```python
from build123d import *

# Parameters (mm, degrees)
F0_W           = 100
F0_H           = 70
F1_DEPTH       = 200
F2_R           = 25
F3_T           = -25
F5_START       = -25
F5_DEPTH       = 50
F6_R           = 24.99999
F9_D           = 25
F9_DEPTH       = 100
F9_TIP         = 7.5107577378
F9_ON_F8_D     = 25
F9_ON_F8_DEPTH = 100
F9_ON_F8_TIP   = 7.5107577378
F10_R          = 15
F11_DEPTH      = 50


# Not quite as in the source:
# - a fillet or chamfer is up to 0.001 mm smaller than in the source, because OpenCascade refuses the exact size


with BuildPart() as f1:
    # F0 (on Front) → F1 (new body)
    with BuildSketch(Plane.XZ):
        with Locations((50, -35)):
            Rectangle(F0_W, F0_H)
    extrude(amount=-F1_DEPTH)

    # F2
    f2_edges = [f1.edges().sort_by_distance(p)[0] for p in [
        (100, 100, -70),
        (0, 100, -70),
        (100, 200, -35),
        (0, 200, -35),
    ]]
    fillet(f2_edges, radius=F2_R)

    # F3
    f3_openings = [f1.faces().sort_by_distance(p)[0] for p in [
        (100, 87.5, -22.5),
        (50, 200, -35),
        (92.67767, 192.67767, -35),
        (7.32233, 192.67767, -35),
        (0, 87.5, -22.5),
        (92.67767, 100, -62.67767),
        (50, 100, -70),
        (7.32233, 100, -62.67767),
    ]]
    offset(amount=F3_T, openings=f3_openings)

    # F4 (on face) → F5 (join)
    with BuildSketch(Plane.YZ.offset(100).offset(F5_START)):
        Polygon((17.6776695297, 17.6776695297), (0, 0), (163, 0), (81.5, 81.5), (28.2842712475, 28.2842712475), (38.8908729653, 17.6776695297), (28.2842712475, 7.0710678119), align=None)
    extrude(amount=-F5_DEPTH)

    # F6 (radius 25 in the source; OpenCascade refuses exactly that, so slightly less here)
    f6_edges = [f1.edges().sort_by_distance(p)[0] for p in [
        (75, 122.25, 40.75),
        (25, 122.25, 40.75),
    ]]
    fillet(f6_edges, radius=F6_R)

    # F9
    with Locations(Plane.XZ):
        with Locations((75, -45), (25, -45)):
            Hole(F9_D / 2, depth=F9_DEPTH)
            with Locations((0, 0, -(F9_DEPTH + F9_TIP / 2))):  # 118° drill point
                Cone(0, F9_D / 2, F9_TIP, mode=Mode.SUBTRACT)

    # F9 on F8
    with Locations(Plane.XY):
        with Locations((75, 175), (25, 175)):
            Hole(F9_ON_F8_D / 2, depth=F9_ON_F8_DEPTH)
            with Locations((0, 0, -(F9_ON_F8_DEPTH + F9_ON_F8_TIP / 2))):  # 118° drill point
                Cone(0, F9_ON_F8_D / 2, F9_ON_F8_TIP, mode=Mode.SUBTRACT)

    # F10 (on face) → F11 (cut)
    with BuildSketch(Plane(origin=(0, 0, 0), x_dir=(1, 0, 0), z_dir=(0, -0.7071067812, 0.7071067812))):
        with Locations((50, 90.2584053334)):
            Circle(F10_R)
    extrude(amount=-F11_DEPTH, mode=Mode.SUBTRACT)


solid = f1.part
```
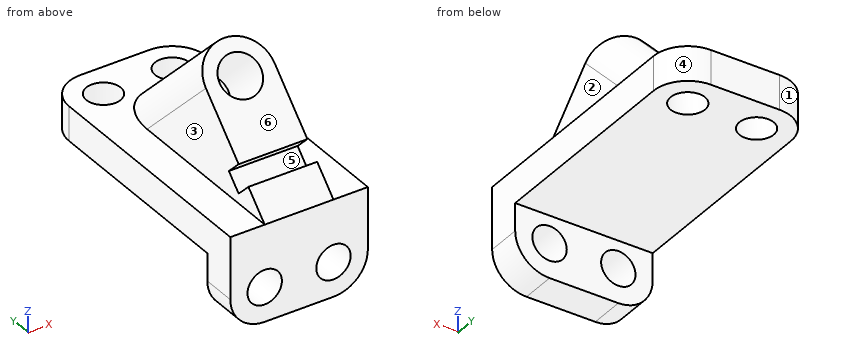
For this review, take the finished solid that the model builds, in its own axes (mm). Face numbers are marked on the shaded views. A direction names the side the tool comes from. Round coordinates to 2 decimals unless told otherwise and drop trailing zeros. Loops run counter-clockwise (first coordinate to the right, second up) from the corner with the lowest first, then second, coordinate; pieces in that order, holes last.
(1) We need section A-A (z = -6.5). Give the boundary of the cut face in (x, y).
Returned:
outline: (0, 0) - (100, 0) - (100, 175) arc R25 ccw to (75, 200) - (25, 200) arc R25 ccw to (0, 175) - close; hole circle Ø25 at (25, 175); hole circle Ø25 at (75, 175)
(2) Clearance check with flat-ended pins moving along their axes: P1, Ø1.5, axis at x = 76, y = 30, coming from the +Z side; P2, Ø13.5, axis at x = 34, z = -37, coming from the +Y side; P3, Ø6, axis at x = 40, y = 76.5, coming from the +Z side. State where each tip first meets the part, or that it passes through.
Returned:
P1: stops at z = 0
P2: stops at y = 25
P3: stops at z = 79.5
(3) We need section D-D (x = 31). Give the boundary of the cut face in (y, z).
Returned:
outline: (0, -70) - (25, -70) - (25, -55.97) - (0, -55.97) - close; (0, -34.03) - (25, -34.03) - (25, -25) - (164.03, -25) - (164.03, 0) - (150.62, 0) - (75.31, 75.31) - (28.28, 28.28) - (38.89, 17.68) - (28.28, 7.07) - (17.68, 17.68) - (0, 0) - close; (185.97, -25) - (200, -25) - (200, 0) - (185.97, 0) - close
(4) We need section C-C (x = 9). Give the boundary of the cut face in (y, z).
Returned:
outline: (0, -64.21) - (25, -64.21) - (25, -25) - (194.21, -25) - (194.21, 0) - (0, 0) - close
(5) Wall thickness on line 1 along Y through (x, z) = (75, -12); line 2 along Z through (x, y) = (29, 161.5); line 3 along Y through (x, z) = (58.5, 7.5): over which ranges is each line inside the solid? List them lowest first.
Returned:
line 1: y = 0 to 162.5, 187.5 to 200
line 2: z = -25 to 0
line 3: y = 7.5 to 27.86, 28.71 to 153.39
(6) Mouldability with a two-part tool opening along Y and no side actions: class the marked faces 4, 5 and 6 as released by +Y, released by -Y, zero draft, split by the parting line, or undercut.
Returned:
face 4: released by +Y
face 5: undercut
face 6: released by -Y
(7) We need section B-B (x = 67.5). Give the boundary of the cut face in (y, z).
Returned:
outline: (0, -70) - (25, -70) - (25, -55) - (0, -55) - close; (0, -35) - (25, -35) - (25, -25) - (165, -25) - (165, 0) - (152.89, 0) - (76.45, 76.45) - (28.28, 28.28) - (38.89, 17.68) - (28.28, 7.07) - (17.68, 17.68) - (0, 0) - close; (185, -25) - (200, -25) - (200, 0) - (185, 0) - close
(8) Tool access review of the marked faces 1, 2 and 3: name each direction out of +Z, -Z, +X, -X, +Y, -Y from which nothing blocks a thin tool from reaching the whole face with its end or side.
Returned:
face 1: +Z, -Z, -X, +Y
face 2: +Z, +X, +Y, -Y
face 3: +Z, -X, +Y, -Y
